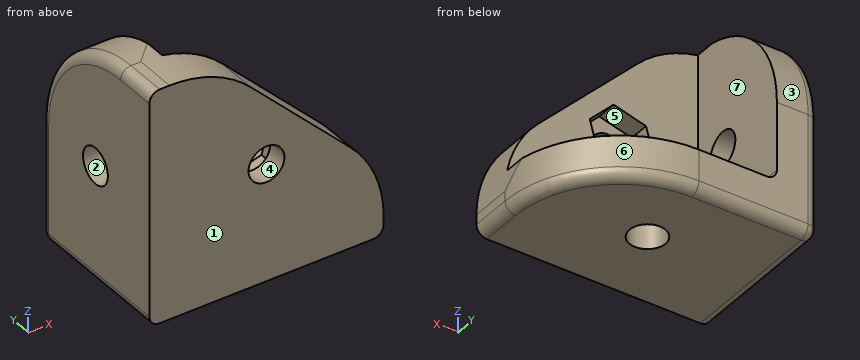
from build123d import *

# Parameters (mm, degrees)
F1_W         = 22.5
F1_H         = 15
F2_DEPTH     = 4
F4_DEPTH     = 18.5
F5_R         = 1.725
F6_DEPTH     = 4
F7_R         = 1.725
F8_DEPTH     = 4
F9_R         = 1.725
F10_DEPTH    = 4
F11_DEPTH    = 2
F12_SIZE     = 16
F13_T1_DEPTH = 59
F13_T3_DEPTH = 59
F13_T5_DEPTH = 26.7817459305
F14_R        = 1


# Not quite as in the source:
# - a fillet or chamfer that OpenCascade refuses, or shapes differently, is made with other operations: its cross-section is extruded or revolved along the edge and cut away or added


with BuildPart() as f2:
    # F1 (on Top) → F2 (new body)
    with BuildSketch(Plane.XY):
        with Locations((11.25, 7.5)):
            Rectangle(F1_W, F1_H)
    extrude(amount=F2_DEPTH)

    # F3 (on face) → F4 (join)
    with BuildSketch(Plane.XY.offset(4)):
        Polygon((4, 15), (0, 15), (0, 0), (22.5, 0), (22.5, 4), (4, 4), align=None)
    extrude(amount=F4_DEPTH)

    # F5 (on face) → F6 (cut, through all)
    with BuildSketch(Plane.XY.offset(4)):
        with Locations((11.25, 7.5)):
            Circle(F5_R)
    extrude(amount=-F6_DEPTH, mode=Mode.SUBTRACT)

    # F7 (on face) → F8 (cut, through all)
    with BuildSketch(Plane.YZ.offset(4)):
        with Locations((7.5, 11.25)):
            Circle(F7_R)
    extrude(amount=-F8_DEPTH, mode=Mode.SUBTRACT)

    # F9 (on face) → F10 (cut, through all)
    with BuildSketch(Plane(origin=(0, 4, 0), x_dir=(-1, 0, 0), z_dir=(0, 1, 0))):
        with Locations((-11.25, 11.25)):
            Circle(F9_R)
    extrude(amount=-F10_DEPTH, mode=Mode.SUBTRACT)

    # F9 (on face) → F11 (cut)
    with BuildSketch(Plane(origin=(0, 4, 0), x_dir=(-1, 0, 0), z_dir=(0, 1, 0))):
        Polygon((-8.1270057994, 10.413196226), (-8.9638095734, 13.5361904266), (-12.086803774, 14.3729942006), (-14.3729942006, 12.086803774), (-13.5361904266, 8.9638095734), (-10.413196226, 8.1270057994), align=None)
        with Locations((-11.25, 11.25)):
            Circle(F9_R, mode=Mode.SUBTRACT)
    extrude(amount=-F11_DEPTH, mode=Mode.SUBTRACT)

    # F12
    f12_edges = [f2.edges().sort_by_distance(p)[0] for p in [
        (22.5, 2, 22.5),
    ]]
    chamfer(f12_edges, length=F12_SIZE)

    # F13: fillet of radius 11 on 4 edges, made by hand

    # F13_s2 → F13_t1 (cut)
    with BuildSketch(Plane.XY.offset(-27.5)):
        with BuildLine():
            ThreePointArc((11.5, 15), (19.2781745931, 11.7781745931), (22.5, 4))
            Line((22.5, 4), (22.5, 15))
            Line((22.5, 15), (11.5, 15))
        make_face()
    extrude(amount=F13_T1_DEPTH, mode=Mode.SUBTRACT)

    # F13_s4 → F13_t3 (cut)
    with BuildSketch(Plane.YZ.offset(-27.5)):
        with BuildLine():
            ThreePointArc((4, 22.5), (11.7781745931, 19.2781745931), (15, 11.5))
            Line((15, 11.5), (15, 22.5))
            Line((15, 22.5), (4, 22.5))
        make_face()
    extrude(amount=F13_T3_DEPTH, mode=Mode.SUBTRACT)

    # F13_s6 → F13_t5 (cut)
    with BuildSketch(Plane.XZ.offset(-15.3908729653)):
        with BuildLine():
            ThreePointArc((1.9436508139, 22.5), (6.1531685699, 21.6626748576), (9.7218254069, 19.2781745931))
            Line((9.7218254069, 19.2781745931), (6.5, 22.5))
            Line((6.5, 22.5), (1.9436508139, 22.5))
        make_face()
        with BuildLine():
            ThreePointArc((19.2781745931, 9.7218254069), (21.6626748576, 6.1531685699), (22.5, 1.9436508139))
            Line((22.5, 1.9436508139), (22.5, 6.5))
            Line((22.5, 6.5), (19.2781745931, 9.7218254069))
        make_face()
    extrude(amount=F13_T5_DEPTH, mode=Mode.SUBTRACT)

    # F14
    f14_edges = [f2.edges().sort_by_distance(p)[0] for p in [
        (0, 2, 22.5),
        (0, 7.5, 0),
        (22.5, 2, 0),
        (4, 9.5, 4),
        (0, 15, 5.75),
        (0, 11.778175, 19.278175),
        (5.75, 15, 0),
        (19.278175, 11.778175, 0),
    ]]
    fillet(f14_edges, radius=F14_R)


solid = f2.part
Design review of the part built by this model. Coordinates are the model's own, in mm. Face numbers are marked on the shaded views. A direction names the side the tool comes from. Round coordinates to 2 decimals unless told otherwise and drop trailing zeros. Write each loop counter-clockwise with the first axis right and the second up, starting at its lowest first coordinate (ties: lowest second). Pieces come first, ordered by that corner, then holes.
Item 1: Draft analysis for pull direction Y (two halves, no side actions). For the marked faces 1, 2, 3 and 4, state which applies: released by +Y, released by -Y, zero draft, split by the parting line, or undercut.
Item 2: For pin 1 Ø3.5 at (x, y) = (17.5, 10.5) entering from +Z; pin 2 Ø9 at (y, z) = (12, 16) entering from +X; pin 3 Ø7 at (x, z) = (12, 11.5) entering from +Y, all flat-tipped, find the tip position at first contact; note any pin that passes through.
Item 3: Consider section B-B on x = 4.5. Give the boundary of the cut face in (y, z).
Item 4: Consider section C-C on y = 7.5. Count the separate pieces of the cut face and the enclosed holes in it, and give its area (3 significant figures).
Item 5: Consider section A-A on z = 2.5. Give the boundary of the cut face in (x, y) (3 decimals).
Item 6: Wall thickness on L1, parallel to Y at x = 11.25, z = 1.25 (3 decimals); L2, parallel to Z at x = 17, y = 12.5; L3, parallel to X at y = 6.5, z = 17: over which ranges is each line inside the solid? List them lowest first.
Item 7: For the marked faces 5, 6 and 7, list the 3-axis set-ups (+Z, -Z, +X, -X, +Y, -Y) from which the entire face can be reached by the end or side of a thin tool; tool diameter is ignored.
Check values:
1. face 1: released by -Y
1. face 2: undercut
1. face 3: released by +Y
1. face 4: zero draft
2. pin 1: stops at z = 4
2. pin 2: stops at x = 4
2. pin 3: stops at y = 4
3. outline: (0, 0) - (14, 0) arc R1 ccw to (15, 1) - (15, 4.13) - (4, 4.13) - (4, 22.2) - (0, 22.2) - close
4. separate pieces: 3
4. enclosed holes: 0
4. area: 131 mm2
5. outline: (0, 0) - (22.486, 0) - (22.486, 4.556) arc R11 ccw to (11.5, 15) - (1, 15) arc R1 ccw to (0, 14) - close; hole circle Ø3.45 at (11.25, 7.5)
6. L1: y = 0 to 5.775, 9.225 to 15
6. L2: z = 0.01 to 4
6. L3: x = 0 to 4
7. face 5: +Y
7. face 6: +Z, -Z, +X, +Y
7. face 7: +Z, +X, +Y
